```python
from build123d import *

# Parameters (mm, degrees)
SKETCH1_R           = 90
SKETCH1_R_2         = 1.5
SKETCH1_W           = 17
SKETCH1_H           = 60
SKETCH1_W_2         = 5
SKETCH1_H_2         = 21
BOSS_EXTRUDE1_DEPTH = 5
SKETCH3_R           = 1.5
OUTER_SCREWS_DEPTH  = 10
SKETCH2_R           = 1.5
SKETCH2_W           = 16
SKETCH2_H           = 8.5
SAFETY_LINK_DEPTH   = 10


with BuildPart() as part:
    # Sketch1 → Boss-Extrude1 (new body)
    with BuildSketch(Plane(origin=(0, 0, 0), x_dir=(1, 0, 0), z_dir=(0, 1, 0))):
        with Locations(Location((0, 0, 0), (0, 0, 270))):
            Circle(SKETCH1_R)
        with Locations(Location((-6, 71, 0), (0, 0, 270))):
            Circle(SKETCH1_R_2, mode=Mode.SUBTRACT)
        with Locations(Location((6, 49, 0), (0, 0, 270))):
            Circle(SKETCH1_R_2, mode=Mode.SUBTRACT)
        with Locations((-57.5, 0)):
            Rectangle(SKETCH1_W, SKETCH1_H, mode=Mode.SUBTRACT)
        with Locations((57.5, 0)):
            Rectangle(SKETCH1_W, SKETCH1_H, mode=Mode.SUBTRACT)
        with Locations((0, 64.5)):
            Rectangle(SKETCH1_W_2, SKETCH1_H_2, mode=Mode.SUBTRACT)
        Polygon((-5.5, 52.5), (0.5, 52.5), (5.789809421, 22.5), (-10.789809421, 22.5), align=None, mode=Mode.SUBTRACT)
    extrude(amount=BOSS_EXTRUDE1_DEPTH)

    # Sketch3 → Outer Screws (cut)
    with BuildSketch(Plane(origin=(0, 5, 0), x_dir=(1, 0, 0), z_dir=(0, 1, 0))):
        with Locations(Location((32.528091751, 78.529760263, 0), (0, 0, 270))):
            Circle(SKETCH3_R)
        with Locations(Location((78.529760263, 32.528091751, 0), (0, 0, 270))):
            Circle(SKETCH3_R)
        with Locations(Location((78.529760263, -32.528091751, 0), (0, 0, 270))):
            Circle(SKETCH3_R)
        with Locations(Location((32.528091751, -78.529760263, 0), (0, 0, 270))):
            Circle(SKETCH3_R)
        with Locations(Location((-32.528091751, -78.529760263, 0), (0, 0, 270))):
            Circle(SKETCH3_R)
        with Locations(Location((-78.529760263, -32.528091751, 0), (0, 0, 270))):
            Circle(SKETCH3_R)
        with Locations(Location((-78.529760263, 32.528091751, 0), (0, 0, 270))):
            Circle(SKETCH3_R)
        with Locations(Location((-32.528091751, 78.529760263, 0), (0, 0, 270))):
            Circle(SKETCH3_R)
    extrude(amount=-OUTER_SCREWS_DEPTH, mode=Mode.SUBTRACT)

    # Sketch2 → Safety Link (cut)
    with BuildSketch(Plane(origin=(0, 5, 0), x_dir=(1, 0, 0), z_dir=(0, 1, 0))):
        with Locations(Location((-12, 0, 0), (0, 0, 270))):
            Circle(SKETCH2_R)
        with Locations(Location((12, 0, 0), (0, 0, 270))):
            Circle(SKETCH2_R)
        Rectangle(SKETCH2_W, SKETCH2_H)
    extrude(amount=-SAFETY_LINK_DEPTH, mode=Mode.SUBTRACT)


solid = part.part
```
Could you check a few things on this model? Use its own coordinates, in mm. A direction names the side the tool comes from. Round coordinates to 2 decimals unless told otherwise and drop trailing zeros. Loops run counter-clockwise (first coordinate to the right, second up) from the corner with the lowest first, then second, coordinate; pieces in that order, holes last. Notation, with made-up numbers: M 27,20.5 L 61,20.5 A37 ccw 61,59.5 Z; hole C 2,75 d1. An arc over 180 degrees is marked long. Write item = value, one per line.
1. Will these pins go through, and if not, where does the flat tip stop? P1, Ø1.5, axis at x = -53.5, y = 2.5, coming from the +Z side; P2, Ø2.5, axis at x = 59.5, y = 3, coming from the -Z side; P3, Ø4, axis at x = 12, z = 0, coming from the -Y side; P4, Ø3, axis at x = -42, y = 2, coming from the -Z side.
Results below:
P1 = 72.92
P2 = -68.61
P3 = 0
P4 = -80.37
2. Thinking about a two-plate mould opening in Z: for faces 3 (the face through (-34.471, 2.465, 83.137)), 4 (the face through (3.108, 2.465, -37.71)), 5 (the face through (1, 0, 19)), which applies, +Z half, -Z half, draft (parallel to the pull), parting line (faces both ways), or undercut?
Results below:
face_3 = parting line
face_4 = undercut
face_5 = draft
3. I want a section at A-A, the plane z = -60. Write out the boundary of the cut face in (x, y).
Results below:
outline = M -67.08,0 L -2.5,0 L -2.5,5 L -67.08,5 Z; M 2.5,0 L 67.08,0 L 67.08,5 L 2.5,5 Z
4. I want a section at B-B, the plane x = -55.5. Write out the boundary of the cut face in (y, z).
Results below:
outline = M 0,-70.85 L 5,-70.85 L 5,-30 L 0,-30 Z; M 0,30 L 5,30 L 5,70.85 L 0,70.85 Z
5. I want a section at D-D, the plane y = 4.1. Count the separate pieces of the cut face and the enclosed holes in it, and give its area (3 significant figures).
Results below:
separate_pieces = 1
enclosed_holes = 17
area = 22,700 mm²
6. I need wall thicknesses on probe 1 along X at (y, z) = (1.8, 0); probe 2 along X at (y, z) = (1.65, -16.5); probe 3 along X at (y, z) = (4.4, 24.5). Which ranges of each line are inside material? Lowest first, please.
Results below:
probe_1 = -90 to -66, -49 to -13.5, -10.5 to -8, 8 to 10.5, 13.5 to 49, 66 to 90
probe_2 = -88.47 to -66, -49 to 49, 66 to 88.47
probe_3 = -86.6 to -66, -49 to 49, 66 to 86.6
7. I want a section at C-C, the plane z = 19. Write out the boundary of the cut face in (x, y), and give its area (3 significant figures).
Results below:
outline = M -87.97,0 L -66,0 L -66,5 L -87.97,5 Z; M -49,0 L 49,0 L 49,5 L -49,5 Z; M 66,0 L 87.97,0 L 87.97,5 L 66,5 Z
area = 710 mm²
8. Which directions (+Z, -Z, +X, -X, +Y, -Y) give clear straight access to the entire face, cutting with the end or side of a thin tool? Please do faces 1 (the face through (-49, 2, 0)), 2 (the face through (1, 5, 19)).
Results below:
face_1 = +Y, -Y
face_2 = +Z, -Z, +X, -X, +Y
